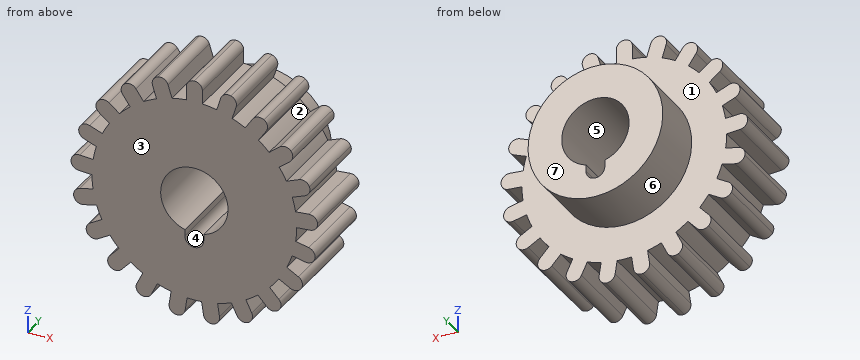
from build123d import *

# Parameters (mm, degrees)
SKETCH_1_R                       = 76
EXTRUDE_1_DEPTH                  = 60
SKETCH_2_R                       = 50
EXTRUDE_2_DEPTH                  = 42
CUT_EXTRUDE_1_DEPTH              = 149.175571536
SKETCH_4_R                       = 7
CUT_EXTRUDE_2_DEPTH              = 149.175571536
EXTRUDE_3_DEPTH                  = 60
FILLET_1_R                       = 6
PATTERN_CIRCULAR_1_COUNT         = 21
FILLET_1_OF_PATTERN_CIRCULAR_1_R = 6


with BuildPart() as part:
    # 草图1 → 凸台-拉伸1 (new body)
    with BuildSketch(Plane(origin=(0, 0, 0), x_dir=(1, 0, 0), z_dir=(0, 1, 0))):
        with Locations(Location((0, 0, 0), (0, 0, 270))):
            Circle(SKETCH_1_R)
    extrude(amount=EXTRUDE_1_DEPTH)

    # 草图2 → 凸台-拉伸2 (add)
    with BuildSketch(Plane(origin=(0, 60, 0), x_dir=(1, 0, 0), z_dir=(0, 1, 0))):
        with Locations(Location((0, 0, 0), (0, 0, 90))):
            Circle(SKETCH_2_R)
    extrude(amount=EXTRUDE_2_DEPTH)

    # 草图3 → 切除-拉伸1 (cut, through all)
    with BuildSketch(Plane(origin=(0, 102, 0), x_dir=(1, 0, 0), z_dir=(0, 1, 0))):
        with BuildLine():
            Line((-7, 24), (-7, 28.8))
            Line((-7, 28.8), (7, 28.8))
            Line((7, 28.8), (7, 24))
            ThreePointArc((7, 24), (0, -25), (-7, 24))
        make_face()
    extrude(amount=-CUT_EXTRUDE_1_DEPTH, mode=Mode.SUBTRACT)

    # 草图4 → 切除-拉伸2 (cut, through all)
    with BuildSketch(Plane(origin=(0, 102, 0), x_dir=(1, 0, 0), z_dir=(0, 1, 0))):
        with Locations((0, 28.8)):
            Circle(SKETCH_4_R)
    extrude(amount=-CUT_EXTRUDE_2_DEPTH, mode=Mode.SUBTRACT)

    # 草图5 → 凸台-拉伸3 (add)
    with BuildSketch(Plane(origin=(0, 0, 0), x_dir=(-1, 0, 0), z_dir=(0, -1, 0))):
        with BuildLine():
            Line((6, -75.7627877), (6, -91.7627877))
            Line((6, -91.7627877), (-6, -91.7627877))
            Line((-6, -91.7627877), (-6, -75.7627877))
            ThreePointArc((-6, -75.7627877), (0, -76), (6, -75.7627877))
        make_face()
    extrude_3 = extrude(amount=-EXTRUDE_3_DEPTH)

    # 圆角1
    fillet_1_edges = [part.edges().sort_by_distance(p)[0] for p in [
        (-6, 30, 91.7627877),
        (6, 30, 91.7627877),
    ]]
    fillet(fillet_1_edges, radius=FILLET_1_R - 0.0001)  # a hair under: the kernel refuses the full size

    # 阵列(圆周)1: 凸台-拉伸3 ×21 about axis
    pattern_circular_1_axis = Axis((0, 0, 0), (0, 1, 0))
    for i in range(1, PATTERN_CIRCULAR_1_COUNT):
        add(extrude_3.rotate(pattern_circular_1_axis, i * 360 / PATTERN_CIRCULAR_1_COUNT))

    # 圆角1 of 阵列(圆周)1
    fillet_1_of_pattern_circular_1_edges = [part.edges().sort_by_distance(p)[0] for p in [
        (21.314119658, 30, 89.454555555),
        (32.780993328, 30, 85.917493462),
        (46.734386249, 30, 79.197893585),
        (56.649251541, 30, 72.438052888),
        (68.002097531, 30, 61.904151216),
        (75.483975154, 30, 52.522173426),
        (83.227524026, 30, 39.109953349),
        (87.611616318, 30, 27.939468365),
        (91.057819772, 30, 12.840664496),
        (91.954580895, 30, 0.874218929),
        (90.797228632, 30, -14.569573748),
        (88.126977424, 30, -26.268708694),
        (82.46890527, 30, -40.685241427),
        (76.46890527, 30, -51.077546272),
        (66.812857766, 30, -63.185846861),
        (58.016235304, 30, -71.347919714),
        (45.220194646, 30, -80.072112514),
        (34.408568231, 30, -85.278717384),
        (19.609518787, 30, -89.843619581),
        (7.743548872, 30, -91.632126775),
        (-7.743548872, 30, -91.632126775),
        (-19.609518787, 30, -89.843619581),
        (-34.408568231, 30, -85.278717384),
        (-45.220194646, 30, -80.072112514),
        (-58.016235304, 30, -71.347919714),
        (-66.812857766, 30, -63.185846861),
        (-76.46890527, 30, -51.077546272),
        (-82.46890527, 30, -40.685241427),
        (-88.126977424, 30, -26.268708694),
        (-90.797228632, 30, -14.569573748),
        (-91.954580895, 30, 0.874218929),
        (-91.057819772, 30, 12.840664496),
        (-87.611616318, 30, 27.939468365),
        (-83.227524026, 30, 39.109953349),
        (-75.483975154, 30, 52.522173426),
        (-68.002097531, 30, 61.904151216),
        (-56.649251541, 30, 72.438052888),
        (-46.734386249, 30, 79.197893585),
        (-32.780993328, 30, 85.917493462),
        (-21.314119658, 30, 89.454555555),
    ]]
    fillet(fillet_1_of_pattern_circular_1_edges, radius=FILLET_1_OF_PATTERN_CIRCULAR_1_R - 0.0001)  # a hair under: the kernel refuses the full size


solid = part.part
Verification items for the finished model (mm, model axes). Face numbers are marked on the shaded views. A direction names the side the tool comes from. Round coordinates to 2 decimals unless told otherwise and drop trailing zeros. Write each loop counter-clockwise with the first axis right and the second up, starting at its lowest first coordinate (ties: lowest second). Pieces come first, ordered by that corner, then holes.
(1) Mould release check, pull along X, two halves, no side actions. Record for the marked faces 4, 5, 6 and 7: pulls with the +X half, pulls with the -X half, needs draft (parallel to the pull), parting line crosses it, or undercut.
Returned:
face 4: undercut
face 5: undercut
face 6: parting line crosses it
face 7: needs draft
(2) Section check A-A (x = -60). Enter the section's corners in (y, z), plus the area to 3 significant figures.
Returned:
outline: (0, -68.63) - (60, -68.63) - (60, -55.84) - (0, -55.84) - close; (0, -46.65) - (60, -46.65) - (60, 55.52) - (0, 55.52) - close
area: 6,900 mm2
(3) Section check B-B (y = 65.5). Enter the section's corners in (x, z).
Returned:
outline: circle Ø100 at (0, 0); hole (-7, -28.8) arc R7 ccw to (7, -28.8) - (7, -24) arc R25 ccw (long way) to (-7, -24) - close
(4) Material ranges on line 1 (Z direction, x = 0, y = 22); line 2 (X direction, y = 34, z = -60.5); line 3 (X direction, y = 79.5, z = 0), recorded low to high.
Returned:
line 1: z = -76 to -35.8, 25 to 91.76
line 2: x = -63.85 to -47.95, -46 to 46, 47.95 to 63.85
line 3: x = -50 to -25, 25 to 50
(5) Section check C-C (z = 18.5). Enter the section's corners in (x, y), plus the area to 3 significant figures.
Returned:
outline: (-73.71, 0) - (-16.82, 0) - (-16.82, 102) - (-46.45, 102) - (-46.45, 60) - (-73.71, 60) - close; (16.82, 0) - (73.71, 0) - (73.71, 60) - (46.45, 60) - (46.45, 102) - (16.82, 102) - close
area: 9,320 mm2
(6) Depth check by flat-ended pin: pin 1 Ø5 at (y, z) = (33, -65) entering from -X; pin 2 Ø5.5 at (y, z) = (46.5, -25.5) entering from +X; pin 3 Ø4 at (x, z) = (27.5, -64.5) entering from +Y. Enter the tip coordinate at first touch or a pass-through.
Returned:
pin 1: stops at x = -64.33
pin 2: stops at x = 88.36
pin 3: stops at y = 60
(7) Access from +Z, -Z, +X, -X, +Y, -Y to the whole of each face (thin tool, end or side, straight path). Record for the marked faces 1, 2 and 3.
Returned:
face 1: +Y
face 2: +Y, -Y
face 3: +Z, -Z, +X, -X, -Y
(8) Section check D-D (z = -8.5). Enter the section's corners in (x, y), plus the area to 3 significant figures.
Returned:
outline: (-75.52, 0) - (-23.51, 0) - (-23.51, 102) - (-49.27, 102) - (-49.27, 60) - (-75.52, 60) - close; (23.51, 0) - (75.52, 0) - (75.52, 60) - (49.27, 60) - (49.27, 102) - (23.51, 102) - close
area: 8,410 mm2
